Autodesk Inventor part; units mm, degrees
ref_plane "YZ Plane" through (0, 0, 0) normal (1, 0, 0) x (0, 1, 0)
ref_plane "XZ Plane" through (0, 0, 0) normal (0, 1, 0) x (-1, 0, 0)
ref_plane "XY Plane" through (0, 0, 0) normal (0, 0, 1) x (1, 0, 0)
sketch "Esboço1" plane through (0, 0, 0) normal (1, 0, 0) x (0, 1, 0)
  line L0 (0, 0) -> (25, 0)
  line L1 (25, 0) -> (25, -10)
  line L2 (25, -10) -> (0, -10)
  line L3 (0, -10) -> (0, 0)
  point P0 (20.25, -5)
  point P1 (4.75, -5)
  dimension "d0" = 25
  dimension "d1" = 10
extrude "Extrusão1" add sketch "Esboço1" along normal blind 1.5
fillet "Arredondamento1" radius 2 1 edges at (0.75, 25, 0)
fillet "Arredondamento2" radius 2 1 edges at (0.75, 25, -10)
fillet "Arredondamento3" radius 2 1 edges at (0.75, 0, 0)
fillet "Arredondamento4" radius 2 1 edges at (0.75, 0, -10)
sketch "Esboço2" plane through (1.5, 0, 0) normal (1, 0, 0) x (0, 0, -1)
  line L0 (8, 25) -> (2, 25)
  line L1 (5, 25) -> (5, 0)
  line L2 (2, 0) -> (8, 0)
  circle A0 centre (5, 5) radius 3.75
  circle A1 centre (5, 20.03) radius 3.75
  point P0 (0, 0)
  dimension "d12" = 4.97
  dimension "d13" = 5
  dimension "d15" = 7.5
  dimension "d16" = 7.5
hole "Furo1" at (1.5, 20.03, -5) at (1.5, 5, -5) direction (-1, 0, 0) diameter 4 depth 2 tip angle 118 countersink diameter 7.5 countersink angle 90
sketch "Esboço3" plane through (1.5, 0, 0) normal (1, 0, 0) x (0, 0, -1)
  arc A0 (8, 0) -> (10, 2) centre (8, 2) ccw
  line L0 (8, 0) -> (2, 0)
  line L1 (2, 0) -> (2, 1)
  line L2 (2, 1) -> (8, 1)
  line L3 (8, 1) -> (8, 0)
  point P0 (0, 0)
  dimension "d24" = 1
  dimension "d25" = 6
extrude "Extrusão2" add sketch "Esboço3" along normal blind 6
fillet "Arredondamento5" radius 2 1 edges at (7.5, 0.5, -8)
fillet "Arredondamento6" radius 2 1 edges at (7.5, 0.5, -2)
pattern_linear "Padrão retangular1" count 2 spacing 24 along (0, 1, 0) of "Extrusão2"
fillet "Arredondamento7" radius 2 1 edges at (7.5, 24.5, -8)
fillet "Arredondamento8" radius 2 1 edges at (7.5, 24.5, -2)
sketch "Esboço4" plane through (0, 25, -2) normal (0, 1, 0) x (1, 0, 0)
  line L0 (1.5, 6) -> (5.5, 6)
  line L1 (1.5, 0) -> (5.5, 0)
  line L2 (7.5, 2) -> (7.5, 4)
  circle A0 centre (4.5, 3) radius 2
  point P0 (0, -2)
  dimension "d37" = 4
extrude "Extrusão3" cut sketch "Esboço4" against normal through all
sketch "Esboço5" plane through (1.5, 0, 0) normal (1, 0, 0) x (0, 0, -1)
  line L0 (6, 25) -> (4, 25)
  line L1 (4, 0) -> (6, 0)
  point P0 (0, 0)
  point P1 (5, 25)
  dimension "d40" = 25
sketch "Esboço6" plane through (1.5, 0, 0) normal (1, 0, 0) x (0, 0, -1)
  point P0 (0, 0)
properties part number "TRILHO LATERAL"
Verification items for the finished model (mm, model axes). A direction names the side the tool comes from. Round coordinates to 2 decimals unless told otherwise and drop trailing zeros. Write each loop counter-clockwise with the first axis right and the second up, starting at its lowest first coordinate (ties: lowest second). Pieces come first, ordered by that corner, then holes. Notation, with made-up numbers: (54.5, 30) - (94.5, 30) arc R16 ccw to (94.5, 45) - close; hole circle Ø1 at (-16, -26.75). An arc over 180 degrees is marked (long way). Answer as a JSON object with one key per item and string values. Group by question number.
Q1. Thickness scan on line 1 (Z direction, x = 4.5, y = 24.3); line 2 (Y direction, x = 1.75, z = -5.5); line 3 (X direction, y = 0.35, z = -5). Record the ranges inside material, lowest first.
Q2. Go/stop test with flat-tipped pins: pin 1 Ø5 at (y, z) = (10.5, -3.5) entering from +X; pin 2 Ø0.5 at (x, y) = (3.5, 0.5) entering from -Z; pin 3 Ø0.5 at (x, y) = (4, 24.5) entering from +Z. Record where each tip stops, or that it passes through.
Q3. Tool access check on faces 5 (the cylindrical face through (0.76, 24.43, -0.6)), 6 (the flat face through (2, 1, -5)), 7 (the flat face through (3.5, 0.5, -8)). Record the directions out of +Z, -Z, +X, -X, +Y, -Y that give a thin tool (end or side, any length) a straight path to the whole face; none if there is none.
Q4. Section check B-B, the plane y = 20.03. Enter the section's corners in (x, z), plus the area to 3 significant figures.
Q5. Section check A-A, the plane x = 1.75. Enter the section's corners in (y, z).
Q6. Section check C-C, the plane z = -5. Enter the section's corners in (x, y), plus the area to 3 significant figures.
Q7. Section check D-D, the plane x = 5. Enter the section's corners in (y, z).
Q8. Mould release check, pull along Z, two halves, no side actions. Record for faces 1 (the flat face through (3.5, 24.5, -2)), 2 (the cylindrical face through (0.76, 0.57, -9.4)), 3 (the cylindrical face through (2.502, 24.507, -5.088)), 4 (the flat face through (2, 24, -5)): released by +Z, released by -Z, zero draft, split by the parting line, or undercut.
Found:
{
 "1": {"line 1": "z = -8 to -7, -3 to -2", "line 2": "y = 0 to 1, 24 to 25", "line 3": "x = 0 to 2.5, 6.5 to 7.5"},
 "2": {"pin 1": "stops at x = 1.5", "pin 2": "stops at z = -8", "pin 3": "stops at z = -2"},
 "3": {"face 5": "+Z, +X, -X, +Y", "face 6": "+Z, -Z, +X", "face 7": "-Z, +X, +Y, -Y"},
 "4": {"outline": "(0, -10) - (1.5, -10) - (1.5, -8.75) - (0, -7.25) - close; (0, -2.75) - (1.5, -1.25) - (1.5, 0) - (0, 0) - close", "area": "6.00 mm^2"},
 "5": {"outline": "(0, -8) - (1, -8) - (1, -2) - (0, -2) - close; (24, -8) - (25, -8) - (25, -2) - (24, -2) - close"},
 "6": {"outline": "(0, 0) - (2.5, 0) - (2.5, 1) - (1.5, 1) - (1.5, 1.25) - (0, 2.75) - close; (0, 7.25) - (1.5, 8.75) - (1.5, 16.28) - (0, 17.78) - close; (0, 22.28) - (1.5, 23.78) - (1.5, 24) - (2.5, 24) - (2.5, 25) - (0, 25) - close; (6.5, 0) - (7.5, 0) - (7.5, 1) - (6.5, 1) - close; (6.5, 24) - (7.5, 24) - (7.5, 25) - (6.5, 25) - close", "area": "23.5 mm^2"},
 "7": {"outline": "(0, -8) - (1, -8) - (1, -6.94) - (0, -6.94) - close; (0, -3.06) - (1, -3.06) - (1, -2) - (0, -2) - close; (24, -8) - (25, -8) - (25, -6.94) - (24, -6.94) - close; (24, -3.06) - (25, -3.06) - (25, -2) - (24, -2) - close"},
 "8": {"face 1": "released by +Z", "face 2": "released by -Z", "face 3": "undercut", "face 4": "zero draft"}
}
